Study the drawing (mm; zero at the part's minimum x, y, z) and answer. A direction names the side the tool comes from. Coordinates: 2 decimals unless noted, no trailing zeros. Write each loop counter-clockwise with the first axis right and the second up, starting at its lowest first coordinate (ties: lowest second). Pieces come first, ordered by that corner, then holes. Notation, with made-up numbers: (61.5, 71) -> (67.5, 71) arc R16 ccw to (67.5, 99) -> close; hole circle Ø6 at (38.5, 36). An arc over 180 degrees is marked (long way). Answer in a Markdown table with one row per item. Add a question column.
Item 1: Section B-B on z = 5.5 is taken. Write down the section's boundary in (x, y) (1 decimal).
Item 2: Which of the six approach directions +Z, -Z, +X, -X, +Y, -Y give full straight-line access (tool end or side, diameter ignored) to the marked faces 5 and 6?
Item 3: Straight lines are drawn through the part: line 1 (X direction, y = 2.5, z = 1.25); line 2 (X direction, y = 7.5, z = 3.75); line 3 (Z direction, x = 6.5, y = 4.5) (1 decimal). For each, find the intervals that lie inside material, in ascending order. Write a range as from..to.
Item 4: For a pull along Y with two mould halves and no side action, classify the marked faces 1, 2, 3 and 4 as +Y half, -Y half, draft (parallel to the pull), parting line (faces both ways), or undercut.
Item 5: Section C-C on y = 7 is taken. Write down the section's boundary in (x, z).
Item 6: Section D-D on x = 4.5 is taken. Write down the section's boundary in (y, z).
Item 7: Section A-A on x = 6.5 is taken. Write down the section's boundary in (y, z).
Item 8: Given pin 1 Ø2 at (y, z) = (10.5, 5) entering from -X; pin 2 Ø2 at (x, z) = (12.5, 8) entering from -Y; pin 3 Ø3 at (y, z) = (5, 4) entering from -X; pin 4 Ø2 at (x, z) = (5, 3) entering from +Y, each flat-ended and moving along its own axis, determine where each tip first touches the part or whether it passes through.
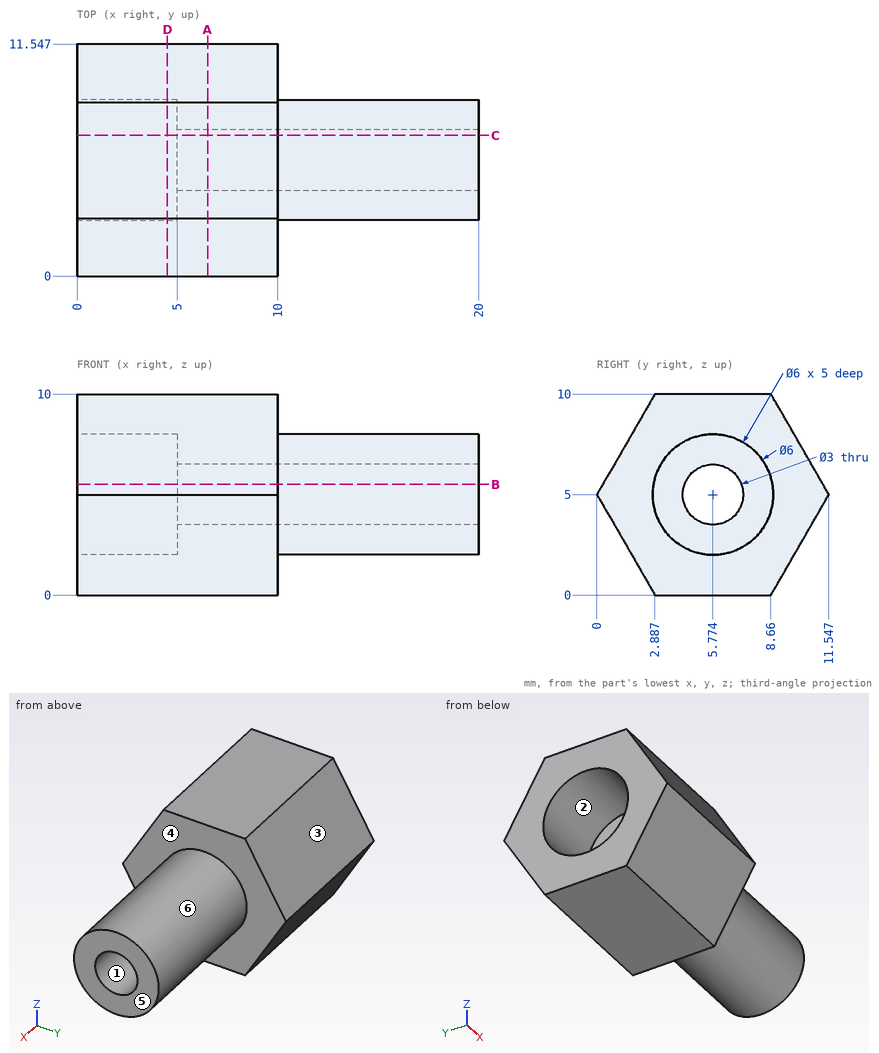
Results below:
| question | item | result |
|---|---|---|
| 1 | outline | (0, 0.3) -> (10, 0.3) -> (10, 2.8) -> (20, 2.8) -> (20, 4.4) -> (5, 4.4) -> (5, 2.8) -> (0, 2.8) -> close; (0, 8.7) -> (5, 8.7) -> (5, 7.2) -> (20, 7.2) -> (20, 8.7) -> (10, 8.7) -> (10, 11.3) -> (0, 11.3) -> close |
| 2 | face 5 | +Z, -Z, +X, +Y, -Y |
| 2 | face 6 | +X |
| 3 | line 1 | x = 0..10 |
| 3 | line 2 | x = 5..20 |
| 3 | line 3 | z = 0..4.2, 5.8..10 |
| 4 | face 1 | undercut |
| 4 | face 2 | undercut |
| 4 | face 3 | +Y half |
| 4 | face 4 | draft |
| 5 | outline | (0, 0) -> (10, 0) -> (10, 2.26) -> (20, 2.26) -> (20, 4.14) -> (5, 4.14) -> (5, 2.26) -> (0, 2.26) -> close; (0, 7.74) -> (5, 7.74) -> (5, 5.86) -> (20, 5.86) -> (20, 7.74) -> (10, 7.74) -> (10, 10) -> (0, 10) -> close |
| 6 | outline | (0, 5) -> (2.89, 0) -> (8.66, 0) -> (11.55, 5) -> (8.66, 10) -> (2.89, 10) -> close; hole circle Ø6 at (5.77, 5) |
| 7 | outline | (0, 5) -> (2.89, 0) -> (8.66, 0) -> (11.55, 5) -> (8.66, 10) -> (2.89, 10) -> close; hole circle Ø3 at (5.77, 5) |
| 8 | pin 1 | stops at x = 0 |
| 8 | pin 2 | stops at y = 3.54 |
| 8 | pin 3 | stops at x = 5 |
| 8 | pin 4 | stops at y = 10.97 |
